Read the model definition and answer for the solid it produces. Units are mm, in the model's axes. Face numbers are marked on the shaded views. Coordinates: 2 decimals unless noted, no trailing zeros. Loops run counter-clockwise (first coordinate to the right, second up) from the corner with the lowest first, then second, coordinate; pieces in that order, holes last. Notation, with made-up numbers: (85.25, -32.75) - (128.25, -32.75) arc R21 ccw to (128.25, 3.25) - close; hole circle Ø2 at (74.5, 40). An arc over 180 degrees is marked (long way). Use CSV: the item, a comma, the result in double quotes.
```python
from build123d import *

# Parameters (mm, degrees)
CROQUIS1_R              = 37.5
CROQUIS1_R_2            = 35
SALIENTE_EXTRUIR1_DEPTH = 15
CROQUIS3_W              = 2
CROQUIS3_H              = 4


with BuildPart() as part:
    # Croquis1 → Saliente-Extruir1 (new body)
    with BuildSketch(Plane(origin=(0, 0, 0), x_dir=(1, 0, 0), z_dir=(0, 1, 0))):
        with Locations((13.541348433, 6.626768313)):
            Circle(CROQUIS1_R)
        with Locations((13.541348433, 6.626768313)):
            Circle(CROQUIS1_R_2, mode=Mode.SUBTRACT)
    extrude(amount=SALIENTE_EXTRUIR1_DEPTH)

    # Barrer1: sweep along a path in Croquis4
    with BuildLine(Plane(origin=(0, -1, 0), x_dir=(-1, 0, 0), z_dir=(0, -1, 0))) as barrer1_path:
        CenterArc((-13.541348433, 6.626768313), 36.25, 0, 360)
    # Croquis3 → Barrer1 (sweep)
    with BuildSketch(Plane.XY.offset(-6.626768313)):
        with Locations((-22.208651567, -1.9)):
            Rectangle(CROQUIS3_W, CROQUIS3_H)
    sweep(path=barrer1_path.line)


solid = part.part
```
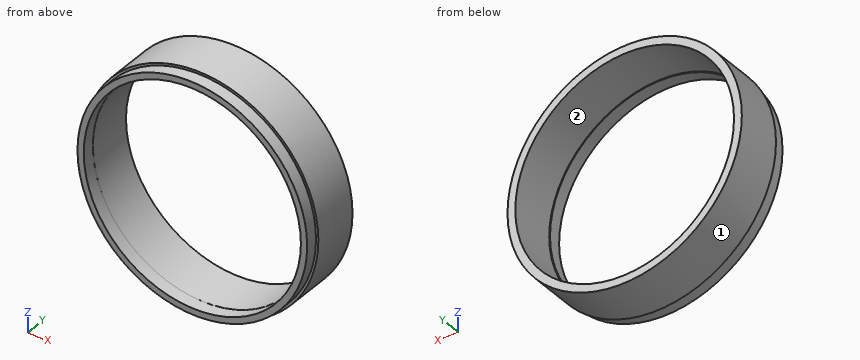
Q1. Find the intervals of material crossed by probe 1 along X at (y, z) = (9, 15); probe 2 along X at (y, z) = (2.25, -25.5); probe 3 along Z at (x, y) = (13, 4), in increasing order. Write a range as [from, to].
Reported:
probe 1,"x = [-17.09, -13.98], [41.06, 44.18]"
probe 2,"x = [-18.86, -15.93], [43.02, 45.95]"
probe 3,"z = [-44.12, -41.62], [28.37, 30.87]"
Q2. The part is cut by section A-A on y = 14. Determine the outline of the cut face in (x, z), and give its area (3 significant figures).
Reported:
outline,"circle Ø75 at (13.54, -6.63); hole circle Ø70 at (13.54, -6.63)"
area,"569 mm²"
Q3. For a pull along X with two mould halves and no side action, classify the marked faces 1 and 2 as +X half, -X half, draft (parallel to the pull), parting line (faces both ways), or undercut.
Reported:
face 1,"parting line"
face 2,"undercut"
Q4. Given P1, Ø10, axis at x = 10, y = 6, coming from the +Z side; P2, Ø2, axis at x = 7.5, y = 8, coming from the +Z side; P3, Ø3, axis at x = -2, y = 7.5, coming from the +Z side, each flat-ended and moving along its own axis, determine where each tip first touches the part or whether it passes through.
Reported:
P1,"stops at z = 30.87"
P2,"stops at z = 30.53"
P3,"stops at z = 28.15"
